```python
from build123d import *

# Parameters (mm, degrees)
SKETCH_2_W           = 40
SKETCH_2_H           = 40
EXTRUDE_1_DEPTH      = 42
CUT_EXTRUDE_1_DEPTH  = 42
CUT_EXTRUDE_START    = 7
SKETCH_5_W           = 35.4
SKETCH_5_H           = 30.8
CUT_EXTRUDE_2_DEPTH  = 42
EXTRUDE_2_DEPTH      = 40
CUT_EXTRUDE_3_REACH  = 81.267
CUT_EXTRUDE_START_2  = -7
SKETCH_7_W           = 31
SKETCH_7_H           = 35.5
CUT_EXTRUDE_4_DEPTH  = 1
CUT_EXTRUDE_5_DEPTH  = 1
SKETCH_14_W          = 31
SKETCH_14_H          = 34.585786438
CUT_EXTRUDE_7_DEPTH  = 34.5
SKETCH_15_R          = 6.5
CUT_EXTRUDE_8_DEPTH  = 10
SKETCH_16_R          = 6.5
CUT_EXTRUDE_9_DEPTH  = 10
SKETCH_17_R          = 8.5
CUT_EXTRUDE_10_DEPTH = 3.5
SKETCH_19_W          = 28
SKETCH_19_H          = 28
SKETCH_19_R          = 6.5
EXTRUDE_3_DEPTH      = 2
SKETCH_20_R          = 8.5
CUT_EXTRUDE_11_DEPTH = 3.5
SKETCH_21_W          = 28
SKETCH_21_H          = 28
SKETCH_21_R          = 6.5
EXTRUDE_4_DEPTH      = 2
EXTRUDE_START        = 0.1
EXTRUDE_5_DEPTH      = 32.6
SKETCH_23_R          = 8.5
EXTRUDE_6_DEPTH      = 1.6
SKETCH_24_W          = 10
SKETCH_24_H          = 4.5
SKETCH_24_W_2        = 4.5
SKETCH_24_H_2        = 10
EXTRUDE_7_DEPTH      = 1.6
SKETCH_25_R          = 8.5
EXTRUDE_8_DEPTH      = 1.6
SKETCH_26_W          = 10
SKETCH_26_H          = 4.5
SKETCH_26_W_2        = 4.5
SKETCH_26_H_2        = 10
EXTRUDE_9_DEPTH      = 1.6


with BuildPart() as part:
    # Эскиз2 → Бобышка-Вытянуть1 (new body)
    with BuildSketch(Plane(origin=(0, 0, 0), x_dir=(1, 0, 0), z_dir=(0, 1, 0))):
        Rectangle(SKETCH_2_W, SKETCH_2_H)
    extrude(amount=EXTRUDE_1_DEPTH)

    # Эскиз4 → Вырез-Вытянуть1 (cut)
    with BuildSketch(Plane.XY.offset(20)):
        Polygon((20, 42), (-20, 42), (20, 25.431457505), align=None)
    extrude(amount=-CUT_EXTRUDE_1_DEPTH, mode=Mode.SUBTRACT)

    # Эскиз5 → Вырез-Вытянуть2 (cut)
    with BuildSketch(Plane(origin=(0, 0, 0), x_dir=(1, 0, 0), z_dir=(0, 1, 0)).offset(CUT_EXTRUDE_START)):
        with Locations((-2.3, 0)):
            Rectangle(SKETCH_5_W, SKETCH_5_H)
    extrude(amount=CUT_EXTRUDE_2_DEPTH, mode=Mode.SUBTRACT)

    # Эскиз6 → Бобышка-Вытянуть2 (add)
    with BuildSketch(Plane.XY.offset(20)):
        Polygon((20, 25.431457505), (38.384776311, 43.816233816), (10.100505063, 72.100505063), (-20, 42), align=None)
    extrude(amount=-EXTRUDE_2_DEPTH)

    # Вырез-Вытянуть3: up to this plane
    cut_extrude_3_end = Plane(origin=(20, 25.431457505, -94.744779783), z_dir=(0.382683432, 0.923879533, 0))
    # Эскиз7 → Вырез-Вытянуть3 (cut, up to the surface)
    with BuildSketch(Plane(origin=(41.100505063, 41.100505063, 0), x_dir=(0, 0, -1), z_dir=(0.707106781, 0.707106781, 0)).offset(CUT_EXTRUDE_START_2), mode=Mode.PRIVATE) as cut_extrude_3_sk1:
        with Locations((0, 26.090620434)):
            Rectangle(SKETCH_7_W, SKETCH_7_H)
    cut_extrude_3_tool1 = split(extrude(cut_extrude_3_sk1.sketch, amount=-CUT_EXTRUDE_3_REACH, mode=Mode.PRIVATE), bisect_by=cut_extrude_3_end, keep=Keep.BOTH, mode=Mode.PRIVATE)
    add(cut_extrude_3_tool1.solids().sort_by_distance((17.701903, 54.599612, 0))[0], mode=Mode.SUBTRACT)

    # Эскиз8 → Вырез-Вытянуть4 (cut)
    with BuildSketch(Plane.ZY.offset(20)):
        Polygon((-16.4, 42), (-16.4, 4), (16.4, 4), (16.4, 42), (15.4, 42), (15.4, 7), (-15.4, 7), (-15.4, 42), align=None)
    extrude(amount=-CUT_EXTRUDE_4_DEPTH, mode=Mode.SUBTRACT)

    # Эскиз12 → Вырез-Вытянуть5 (cut)
    with BuildSketch(Plane(origin=(-31, 31, 0), x_dir=(0, 0, 1), z_dir=(-0.707106781, 0.707106781, 0))):
        Polygon((-16.4, 15.556349186), (-16.4, 54.124891681), (16.4, 54.124891681), (16.4, 15.556349186), (15.5, 15.556349186), (15.5, 51.124891681), (-15.5, 51.124891681), (-15.5, 15.556349186), align=None)
    extrude(amount=-CUT_EXTRUDE_5_DEPTH, mode=Mode.SUBTRACT)

    # Эскиз14 → Вырез-Вытянуть7 (cut)
    with BuildSketch(Plane.ZY.offset(19)):
        with Locations((0, 24.292893219)):
            Rectangle(SKETCH_14_W, SKETCH_14_H)
    extrude(amount=-CUT_EXTRUDE_7_DEPTH, mode=Mode.SUBTRACT)

    # Эскиз15 → Вырез-Вытянуть8 (cut)
    with BuildSketch(Plane(origin=(41.100505063, 41.100505063, 0), x_dir=(0, 0, -1), z_dir=(0.707106781, 0.707106781, 0))):
        with Locations(Location((0, 23.840620434, 0), (0, 0, 90))):  # turned: the seam where the file's is
            Circle(SKETCH_15_R)
    extrude(amount=-CUT_EXTRUDE_8_DEPTH, mode=Mode.SUBTRACT)

    # Эскиз16 → Вырез-Вытянуть9 (cut)
    with BuildSketch(Plane.XZ):
        with Locations(Location((0, 0, 0), (0, 0, 270))):  # turned: the seam where the file's is
            Circle(SKETCH_16_R)
    extrude(amount=-CUT_EXTRUDE_9_DEPTH, mode=Mode.SUBTRACT)

    # Эскиз17 → Вырез-Вытянуть10 (cut)
    with BuildSketch(Plane(origin=(41.100505063, 41.100505063, 0), x_dir=(0, 0, -1), z_dir=(0.707106781, 0.707106781, 0))):
        Polygon((0, 42.840620434), (-5, 42.840620434), (-5, 36.840620434), (-13, 28.840620434), (-19, 28.840620434), (-19, 23.840620434), (-19, 18.840620434), (-13, 18.840620434), (-5, 10.840620434), (-5, 4.840620434), (5, 4.840620434), (5, 10.840620434), (13, 18.840620434), (19, 18.840620434), (19, 28.840620434), (13, 28.840620434), (5, 36.840620434), (5, 42.840620434), align=None)
        with Locations(Location((0, 23.840620434, 0), (0, 0, 90))):  # turned: the seam where the file's is
            Circle(SKETCH_17_R, mode=Mode.SUBTRACT)
    extrude(amount=-CUT_EXTRUDE_10_DEPTH, mode=Mode.SUBTRACT)

    # Эскиз19 → Бобышка-Вытянуть3 (add)
    with BuildSketch(Plane(origin=(38.625631329, 38.625631329, 0), x_dir=(0, 0, -1), z_dir=(0.707106781, 0.707106781, 0))):
        with Locations((0, 23.840620434)):
            Rectangle(SKETCH_19_W, SKETCH_19_H)
        with Locations(Location((0, 23.840620434, 0), (0, 0, 90))):  # turned: the seam where the file's is
            Circle(SKETCH_19_R, mode=Mode.SUBTRACT)
    extrude(amount=EXTRUDE_3_DEPTH)

    # Эскиз20 → Вырез-Вытянуть11 (cut)
    with BuildSketch(Plane.XZ):
        Polygon((0, 19), (-5, 19), (-5, 13), (-13, 5), (-19, 5), (-19, 0), (-19, -5), (-13, -5), (-5, -13), (-5, -19), (5, -19), (5, -13), (13, -5), (19, -5), (19, 5), (13, 5), (5, 13), (5, 19), align=None)
        with Locations(Location((0, 0, 0), (0, 0, 270))):  # turned: the seam where the file's is
            Circle(SKETCH_20_R, mode=Mode.SUBTRACT)
    extrude(amount=-CUT_EXTRUDE_11_DEPTH, mode=Mode.SUBTRACT)

    # Эскиз21 → Бобышка-Вытянуть4 (add)
    with BuildSketch(Plane.XZ.offset(-3.5)):
        Rectangle(SKETCH_21_W, SKETCH_21_H)
        with Locations(Location((0, 0, 0), (0, 0, 270))):  # turned: the seam where the file's is
            Circle(SKETCH_21_R, mode=Mode.SUBTRACT)
    extrude(amount=EXTRUDE_4_DEPTH)

    # Эскиз22 → Бобышка-Вытянуть5 (add)
    with BuildSketch(Plane(origin=(0, 0, 16.4), x_dir=(-1, 0, 0), z_dir=(0, 0, -1)).offset(EXTRUDE_START)):
        Polygon((-7.908474042, 68.494260479), (-7.201367261, 69.201367261), (20, 42), (20, 4.1), (19, 4.1), (19, 41.585786438), align=None)
    extrude(amount=EXTRUDE_5_DEPTH)

    # Эскиз23 → Бобышка-Вытянуть6 (add)
    with BuildSketch(Plane(origin=(40.039844892, 40.039844892, 0), x_dir=(0, 0, -1), z_dir=(0.707106781, 0.707106781, 0))):
        Polygon((-19, 18.840620434), (-19, 28.840620434), (-13, 28.840620434), (-5, 36.840620434), (-5, 42.840620434), (5, 42.840620434), (5, 36.840620434), (13, 28.840620434), (19, 28.840620434), (19, 18.840620434), (13, 18.840620434), (5, 10.840620434), (5, 4.840620434), (-5, 4.840620434), (-5, 10.840620434), (-13, 18.840620434), align=None)
        with Locations(Location((0, 23.840620434, 0), (0, 0, 270))):  # turned: the seam where the file's is
            Circle(SKETCH_23_R, mode=Mode.SUBTRACT)
    extrude(amount=EXTRUDE_6_DEPTH)

    # Эскиз24 → Бобышка-Вытянуть7 (add)
    with BuildSketch(Plane(origin=(41.171215742, 41.171215742, 0), x_dir=(0, 0, -1), z_dir=(0.707106781, 0.707106781, 0))):
        with Locations((0, 40.590620434)):
            Rectangle(SKETCH_24_W, SKETCH_24_H)
        with Locations((-16.75, 23.840620434)):
            Rectangle(SKETCH_24_W_2, SKETCH_24_H_2)
        with Locations((0, 7.090620434)):
            Rectangle(SKETCH_24_W, SKETCH_24_H)
        with Locations((16.75, 23.840620434)):
            Rectangle(SKETCH_24_W_2, SKETCH_24_H_2)
    extrude(amount=EXTRUDE_7_DEPTH)

    # Эскиз25 → Бобышка-Вытянуть8 (add)
    with BuildSketch(Plane.XZ.offset(-1.5)):
        Polygon((-5, 13), (-5, 19), (5, 19), (5, 13), (13, 5), (19, 5), (19, -5), (13, -5), (5, -13), (5, -19), (-5, -19), (-5, -13), (-13, -5), (-19, -5), (-19, 5), (-13, 5), align=None)
        with Locations(Location((0, 0, 0), (0, 0, 90))):  # turned: the seam where the file's is
            Circle(SKETCH_25_R, mode=Mode.SUBTRACT)
    extrude(amount=EXTRUDE_8_DEPTH)

    # Эскиз26 → Бобышка-Вытянуть9 (add)
    with BuildSketch(Plane.XZ.offset(0.1)):
        with Locations((0, 16.75)):
            Rectangle(SKETCH_26_W, SKETCH_26_H)
        with Locations((16.75, 0)):
            Rectangle(SKETCH_26_W_2, SKETCH_26_H_2)
        with Locations((0, -16.75)):
            Rectangle(SKETCH_26_W, SKETCH_26_H)
        with Locations((-16.75, 0)):
            Rectangle(SKETCH_26_W_2, SKETCH_26_H_2)
    extrude(amount=EXTRUDE_9_DEPTH)


solid = part.part
```
Here's how the part is built. I have some questions about the finished solid (model axes, mm). A direction names the side the tool comes from. Coordinates: 2 decimals unless noted, no trailing zeros. Order: outer loops, then holes, each group sorted by start corner. A loop starts at its lowest first (then second) coordinate and runs counter-clockwise, first axis right, second up.
1) Which directions (+Z, -Z, +X, -X, +Y, -Y) give clear straight access to the entire face, cutting with the end or side of a thin tool? Please do faces 1 (the face through (0, -1, -19)), 2 (the face through (-14.5, -1, 0)), 3 (the face through (7, -0.1, -6)), 4 (the face through (-1, 32, 15.5)).
2) We'd pull the mould along Y, two halves only. Please class faces 5 (the face through (37.266, 47.339, 0.07)), 6 (the face through (15.5, 17, 0)), 7 (the face through (25, 59, 19)): +Y half, -Y half, draft (parallel to the pull), parting line (faces both ways), or undercut.
3) Imagine slicing it at A-A on z = 0. State how many separate pieces and enclosed holes the cut face has, and give its area (3 significant figures).
4) Will these pins go through, and if not, where does the flat tip stop? pin 1 (14.5 mm diameter, centred on x = 4.5, z = 2.5, fed in from -Y); pin 2 (0.8 mm diameter, centred on x = 0.5, y = -0.5, fed in from -Z); pin 3 (2.5 mm diameter, centred on x = 0, z = 17, fed in from +Y).
5) I need wall thicknesses on line 1 (X direction, y = 5, z = 0); line 2 (Z direction, x = 17.5, y = 35). Which ranges of each line are inside material? Lowest first, please.
6) Imagine slicing it at B-B on y = 39.5. List the corners of the cut face in (x, z) for me, and give its area (3 significant figures).
Response values:
1. face 1: -Z, +X, -X, -Y
1. face 2: +Z, -Z, -Y
1. face 3: -Y
1. face 4: none
2. face 5: +Y half
2. face 6: undercut
2. face 7: draft
3. separate pieces: 2
3. enclosed holes: 4
3. area: 618 mm2
4. pin 1: stops at y = -0.1
4. pin 2: stops at z = -19
4. pin 3: stops at y = 63.25
5. line 1: x = -20 to -6.5, 6.5 to 20
5. line 2: z = -20 to -15.5, 15.5 to 20
6. outline: (-20, -20) - (34.07, -20) - (34.07, 20) - (-20, 20) - (-20, 16.4) - (-19, 16.4) - (-19, 16.3) - (-20, 16.3) - (-20, -16.3) - (-19, -16.3) - (-19, -16.4) - (-20, -16.4) - close; hole (-19, -15.5) - (27.7, -15.5) - (27.7, 15.5) - (-19, 15.5) - close
6. area: 715 mm2
